The listing builds one solid part. Answer for the finished solid, in the listing's coordinates (mm). A direction names the side the tool comes from. Coordinates: 2 decimals unless noted, no trailing zeros. Loops run counter-clockwise (first coordinate to the right, second up) from the corner with the lowest first, then second, coordinate; pieces in that order, holes last. Notation, with made-up numbers: M 89.5,37.25 L 116.5,37.25 A21 cw 116.5,41.25 Z; hole C -38,85 d8. An arc over 180 degrees is marked long. Return JSON: item names as keys, results as strings. Group by question number.
1. Section A-A (z = 0) is taken. Write down the section's boundary in (x, y).
2. Section C-C (x = 2) is taken. Write down the section's boundary in (y, z), then the cut area to 3 significant figures.
3. Section D-D (x = 10.75) is taken. Write down the section's boundary in (y, z).
4. Straight lines are drawn through the part: L1, parallel to Y at x = 5, z = 0; L2, parallel to Y at x = 3, z = 0; L3, parallel to Z at x = 7.25, y = 3.75. For each, find the intervals that lie inside material, in ascending order. Write a range as from..to.
5. The mould has two halves that part along Y. Classify faces 1 (the face through (1.97, -0.08, 23.75)), 2 (the face through (2, 0, 21)), 3 (the face through (1.97, -8.34, -13.53)), 4 (the face through (1.97, 8.44, -13.33)): pulls with the +Y half, pulls with the -Y half, needs draft (parallel to the pull), parting line crosses it, or undercut.
6. Which of the six approach directions +Z, -Z, +X, -X, +Y, -Y give full straight-line access (tool end or side, diameter ignored) to faces 5 (the face through (5.97, 2.99, -9.51)), 6 (the face through (6.34, -4.88, 1.08))?
7. Given P1, Ø2, axis at y = 5, z = -9, coming from the +X side; P2, Ø6, axis at y = 0, z = -18.5, coming from the +X side; P3, Ø6.5, axis at y = 0, z = 18.5, coming from the -X side; P4, Ø3, axis at x = 1.5, y = -4, coming from the -Z side, each flat-ended and moving along its own axis, determine where each tip first touches the part or whether it passes through.
8. Section B-B (y = 0) is taken. Write down the section's boundary in (x, z), then the cut area to 3 significant figures.
```python
from build123d import *

# Parameters (mm, degrees)
SKETCH1_R           = 2.5
BOSS_EXTRUDE1_DEPTH = 4
SKETCH2_R           = 9.969747688
BOSS_EXTRUDE2_DEPTH = 4
SKETCH3_R           = 6
BOSS_EXTRUDE3_DEPTH = 4.5
SKETCH4_R           = 5
CUT_EXTRUDE1_DEPTH  = 31.042677977


with BuildPart() as part:
    # Sketch1 → Boss-Extrude1 (new body)
    with BuildSketch(Plane(origin=(0, 0, 0), x_dir=(0, 0, -1), z_dir=(1, 0, 0))):
        with BuildLine():
            Line((-20.841216216, 4.699064442), (-6.02027027, 12.083308565))
            ThreePointArc((-6.02027027, 12.083308565), (0, 13.5), (6.02027027, 12.083308565))
            Line((6.02027027, 12.083308565), (20.841216216, 4.699064442))
            ThreePointArc((20.841216216, 4.699064442), (23.75, 0), (20.841216216, -4.699064442))
            Line((20.841216216, -4.699064442), (6.02027027, -12.083308565))
            ThreePointArc((6.02027027, -12.083308565), (0, -13.5), (-6.02027027, -12.083308565))
            Line((-6.02027027, -12.083308565), (-20.841216216, -4.699064442))
            ThreePointArc((-20.841216216, -4.699064442), (-23.75, 0), (-20.841216216, 4.699064442))
        make_face()
        with Locations((-18.5, 0)):
            Circle(SKETCH1_R, mode=Mode.SUBTRACT)
        with Locations(Location((18.5, 0, 0), (0, 0, 180))):
            Circle(SKETCH1_R, mode=Mode.SUBTRACT)
    extrude(amount=BOSS_EXTRUDE1_DEPTH)

    # Sketch2 → Boss-Extrude2 (add)
    with BuildSketch(Plane(origin=(4, 0, 0), x_dir=(0, 0, -1), z_dir=(1, 0, 0))):
        Circle(SKETCH2_R)
    extrude(amount=BOSS_EXTRUDE2_DEPTH)

    # Sketch3 → Boss-Extrude3 (add)
    with BuildSketch(Plane(origin=(8, 0, 0), x_dir=(0, 0, -1), z_dir=(1, 0, 0))):
        Circle(SKETCH3_R)
    extrude(amount=BOSS_EXTRUDE3_DEPTH)

    # Sketch4 → Cut-Extrude1 (cut, through all)
    with BuildSketch(Plane(origin=(12.5, 0, 0), x_dir=(0, 0, -1), z_dir=(1, 0, 0))):
        Circle(SKETCH4_R)
    extrude(amount=-CUT_EXTRUDE1_DEPTH, mode=Mode.SUBTRACT)


solid = part.part
```
Worked out:
{
 "1": {"outline": "M 0,-13.5 L 4,-13.5 L 4,-9.97 L 8,-9.97 L 8,-6 L 12.5,-6 L 12.5,-5 L 0,-5 Z; M 0,5 L 12.5,5 L 12.5,6 L 8,6 L 8,9.97 L 4,9.97 L 4,13.5 L 0,13.5 Z"},
 "2": {"outline": "M -12.08,-6.02 L -4.7,-20.84 A5.25 ccw 4.7,-20.84 L 12.08,-6.02 A13.5 ccw 12.08,6.02 L 4.7,20.84 A5.25 ccw -4.7,20.84 L -12.08,6.02 A13.5 ccw Z; hole C 0,0 d10; hole C 0,-18.5 d5; hole C 0,18.5 d5", "area": "733 mm^2"},
 "3": {"outline": "C 0,0 d12; hole C 0,0 d10"},
 "4": {"L1": "-9.97..-5, 5..9.97", "L2": "-13.5..-5, 5..13.5", "L3": "-9.24..-3.31, 3.31..9.24"},
 "5": {"face 1": "parting line crosses it", "face 2": "undercut", "face 3": "pulls with the -Y half", "face 4": "pulls with the +Y half"},
 "6": {"face 5": "+X", "face 6": "+X, -X"},
 "7": {"P1": "x = 8", "P2": "x = 4", "P3": "x = 0", "P4": "z = -23.12"},
 "8": {"outline": "M 0,-23.75 L 4,-23.75 L 4,-21 L 0,-21 Z; M 0,-16 L 4,-16 L 4,-9.97 L 8,-9.97 L 8,-6 L 12.5,-6 L 12.5,-5 L 0,-5 Z; M 0,5 L 12.5,5 L 12.5,6 L 8,6 L 8,9.97 L 4,9.97 L 4,16 L 0,16 Z; M 0,21 L 4,21 L 4,23.75 L 0,23.75 Z", "area": "159 mm^2"}
}
